Input: dimensioned drawing with shaded views. Units: mm. Origin: part minimum x, y, z. A direction names the side the tool comes from. Round coordinates to 2 decimals unless told otherwise and drop trailing zeros. Loops run counter-clockwise (first coordinate to the right, second up) from the corner with the lowest first, then second, coordinate; pieces in that order, holes last.
1) Ray query, line 1 along Z through (x, y) = (16.5, 26); line 2 along Y through (x, z) = (5.5, 6.3); line 3 along Y through (x, z) = (17, 30.5). Return the intervals inside material, ascending.
2) Access query for the marked faces 4, 5 and 6. Directions: +Z, -Z, +X, -X, +Y, -Y. A direction counts if a zero-diameter tool reaches every point of the face in a straight line with its end or side. Return the directions, or none.
3) Section B-B, the plane x = 32. Return loops of the section in (y, z), and give its area (3 significant figures).
4) Section D-D, the plane y = 11. Return loops of the section in (x, z), and give its area (3 significant figures).
5) Draft query along X for the marked faces 1, 2 and 3. Return one class per face: pulls with the +X half, pulls with the -X half, needs draft (parallel to the pull), parting line crosses it, or undercut.
6) Section C-C, the plane z = 25. Return loops of the section in (x, y).
7) Section A-A, the plane z = 40. Return loops of the section in (x, y), and give its area (3 significant figures).
8) First-contact query: pin 1 (1 mm diameter, centred on x = 26, z = 5, fed in from -Y); pin 2 (1 mm diameter, centred on x = 21, y = 27, fed in from -Z); pin 3 (8 mm diameter, centred on y = 26.5, z = 18.5, fed in from -X); pin 4 (11 mm diameter, centred on x = 4.5, y = 11.5, fed in from +Z). Flat tips, straight axial feed; report the tip coordinate or a pass-through.
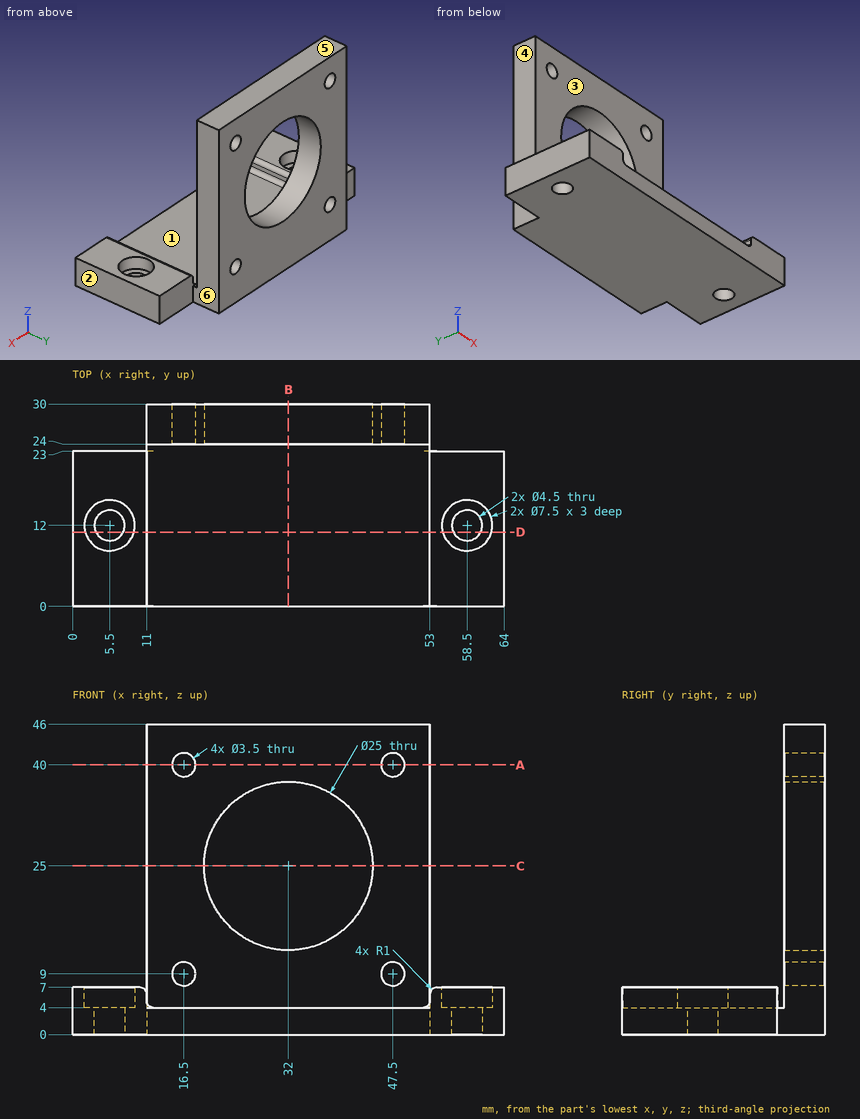
Final values:
1. line 1: z = 0 to 7.25, 10.75 to 38.25, 41.75 to 46
1. line 2: y = 0 to 8.25, 15.75 to 23
1. line 3: y = 24 to 30
2. face 4: +Z, -Z, -X, +Y
2. face 5: +Z, +X, -X, +Y, -Y
2. face 6: +Z, -Z, +X, +Y
3. outline: (0, 0) - (30, 0) - (30, 12.5) - (24, 12.5) - (24, 4) - (0, 4) - close; (24, 37.5) - (30, 37.5) - (30, 46) - (24, 46) - close
3. area: 222 mm2
4. outline: (0, 0) - (3.48, 0) - (3.48, 4) - (1.89, 4) - (1.89, 7) - (0, 7) - close; (7.52, 0) - (56.48, 0) - (56.48, 4) - (54.89, 4) - (54.89, 7) - (54, 7) arc R1 ccw to (53, 6) - (53, 5) arc R1 cw to (52, 4) - (12, 4) arc R1 cw to (11, 5) - (11, 6) arc R1 ccw to (10, 7) - (9.11, 7) - (9.11, 4) - (7.52, 4) - close; (60.52, 0) - (64, 0) - (64, 7) - (62.11, 7) - (62.11, 4) - (60.52, 4) - close
4. area: 246 mm2
5. face 1: undercut
5. face 2: pulls with the +X half
5. face 3: needs draft
6. outline: (11, 24) - (19.5, 24) - (19.5, 30) - (11, 30) - close; (44.5, 24) - (53, 24) - (53, 30) - (44.5, 30) - close
7. outline: (11, 24) - (14.75, 24) - (14.75, 30) - (11, 30) - close; (18.25, 24) - (45.75, 24) - (45.75, 30) - (18.25, 30) - close; (49.25, 24) - (53, 24) - (53, 30) - (49.25, 30) - close
7. area: 210 mm2
8. pin 1: stops at y = 24
8. pin 2: stops at z = 0
8. pin 3: stops at x = 11
8. pin 4: stops at z = 7
